Here's how the part is built. I have some questions about the finished solid (model axes, mm). Face numbers are marked on the shaded views. A direction names the side the tool comes from. Coordinates: 2 decimals unless noted, no trailing zeros. Order: outer loops, then holes, each group sorted by start corner. A loop starts at its lowest first (then second) coordinate and runs counter-clockwise, first axis right, second up. Notation, with made-up numbers: (-27, 54.5) - (29, 54.5) arc R19 cw to (29, 66.5) - close; hole circle Ø5 at (71.25, 87.25). An arc over 180 degrees is marked (long way). Answer in a Markdown table with one row per item. Add a question column.
Item 1: I want a section at A-A (z = 5.5). Please give me the cut outline in (x, y) (3 decimals).
Item 2: On a 3-axis mill with a long thin cutter (end or side, diameter ignored), from which of +Z, -Z, +X, -X, +Y, -Y can I reach the whole of each face in a straight line? I mean the marked faces 5, 6, 7 and 8. Say none if no direction works.
Item 3: Thinking about a two-plate mould opening in X: for the marked faces 1, 2, 3 and 4, which applies, +X half, -X half, draft (parallel to the pull), parting line (faces both ways), or undercut?
Item 4: Will these pins go through, and if not, where does the flat tip stop? pin 1 Ø4 at (x, z) = (19.5, 38) entering from -Y (3 decimals); pin 2 Ø2.5 at (y, z) = (-11, 63.5) entering from -X (3 decimals); pin 3 Ø18 at (x, y) = (-3, -55.5) entering from +Z (3 decimals).
Item 5: I want a section at B-B (y = -44.5). Please give me the cut outline in (x, z) (3 decimals).
Item 6: If I drill on line 1 along Y through (x, z) = (83.5, 46) (3 decimals); line 2 along X through (y, z) = (-36, 39) (3 decimals); line 3 along X through (y, z) = (-48, -2) (3 decimals), over which ranges is the centre line in solid material (lowest first)? Write a range as from..to.
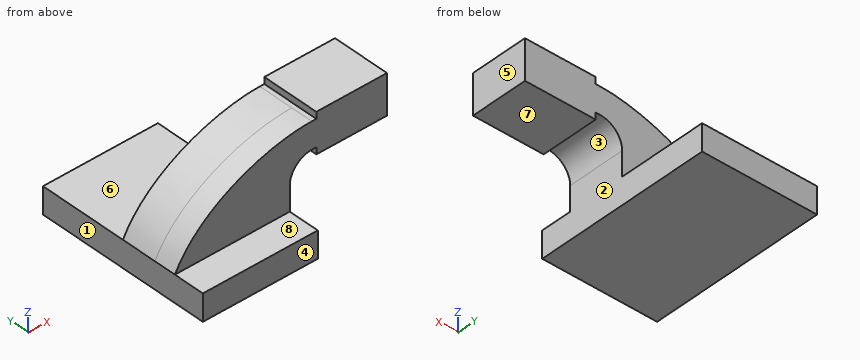
```python
from build123d import *

# Parameters (mm, degrees)
F1_DEPTH = 63.5
F0_W     = 25.4
F0_H     = 19.05
F0_H_2   = 4.7498
F0_H_3   = 4.7752
F2_DEPTH = 25.4
F3_DEPTH = 15.875


with BuildPart() as f1:
    # F0 (on Front) → F1 (new body, symmetric)
    with BuildSketch(Plane.XZ):
        Polygon((-41.275, -9.525), (41.275, -9.525), (41.275, 9.525), (22.225, 9.525), (-41.275, 9.525), align=None)
    extrude(amount=F1_DEPTH, both=True)

    # F0 (on Front) → F2 (join)
    with BuildSketch(Plane.XZ):
        Polygon((-41.275, -9.525), (41.275, -9.525), (41.275, 9.525), (22.225, 9.525), (-41.275, 9.525), align=None)
        with BuildLine():
            Line((22.225, 9.525), (41.275, 9.525))
            Line((41.275, 9.525), (41.275, 27.0002))
            ThreePointArc((41.275, 27.0002), (45.9246798487, 38.2255201513), (57.15, 42.8752))
            Line((57.15, 42.8752), (60.325, 42.8752))
            Line((60.325, 42.8752), (60.325, 61.9252))
            Line((60.325, 61.9252), (57.15, 61.9252))
            ThreePointArc((57.15, 61.9252), (32.4542956671, 51.6959043329), (22.225, 27.0002))
            Line((22.225, 27.0002), (22.225, 9.525))
        make_face()
        with BuildLine():
            add(Edge.make_bspline(
                [(-41.275, 9.525), (-23.4616156667, 44.3730577827), (24.9917246401, 62.0542801917), (57.15, 61.9252)],
                knots=[0, 0, 0, 0, 111.5045361635, 111.5045361635, 111.5045361635, 111.5045361635], degree=3))
            Line((-41.275, 9.525), (22.225, 9.525))
            Line((22.225, 9.525), (22.225, 27.0002))
            ThreePointArc((22.225, 27.0002), (32.4542956671, 51.6959043329), (57.15, 61.9252))
        make_face()
        with Locations((73.025, 52.4002)):
            Rectangle(F0_W, F0_H)
        with Locations((73.025, 64.3001)):
            Rectangle(F0_W, F0_H_2)
        with Locations((73.025, 40.4876)):
            Rectangle(F0_W, F0_H_3)
        Polygon((85.725, 66.675), (85.725, 61.9252), (85.725, 42.8752), (85.725, 38.1), (111.125, 38.1), (111.125, 66.675), align=None)
    extrude(amount=F2_DEPTH)

    # F0 (on Front) + F2_face (on face) → F3 (join)
    with BuildSketch(Plane.XZ):
        Polygon((-41.275, -9.525), (41.275, -9.525), (41.275, 9.525), (22.225, 9.525), (-41.275, 9.525), align=None)
        with BuildLine():
            Line((22.225, 9.525), (41.275, 9.525))
            Line((41.275, 9.525), (41.275, 27.0002))
            ThreePointArc((41.275, 27.0002), (45.9246798487, 38.2255201513), (57.15, 42.8752))
            Line((57.15, 42.8752), (60.325, 42.8752))
            Line((60.325, 42.8752), (60.325, 61.9252))
            Line((60.325, 61.9252), (57.15, 61.9252))
            ThreePointArc((57.15, 61.9252), (32.4542956671, 51.6959043329), (22.225, 27.0002))
            Line((22.225, 27.0002), (22.225, 9.525))
        make_face()
        with BuildLine():
            add(Edge.make_bspline(
                [(-41.275, 9.525), (-23.4616156667, 44.3730577827), (24.9917246401, 62.0542801917), (57.15, 61.9252)],
                knots=[0, 0, 0, 0, 111.5045361635, 111.5045361635, 111.5045361635, 111.5045361635], degree=3))
            Line((-41.275, 9.525), (22.225, 9.525))
            Line((22.225, 9.525), (22.225, 27.0002))
            ThreePointArc((22.225, 27.0002), (32.4542956671, 51.6959043329), (57.15, 61.9252))
        make_face()
        with Locations((73.025, 52.4002)):
            Rectangle(F0_W, F0_H)
        with Locations((73.025, 64.3001)):
            Rectangle(F0_W, F0_H_2)
        with Locations((73.025, 40.4876)):
            Rectangle(F0_W, F0_H_3)
        Polygon((85.725, 66.675), (85.725, 61.9252), (85.725, 42.8752), (85.725, 38.1), (111.125, 38.1), (111.125, 66.675), align=None)
    with BuildSketch(Plane(origin=(36.4198277408, -25.4, 38.4190839989), x_dir=(1, 0, 0), z_dir=(0, -1, 0))):
        with BuildLine():
            add(Edge.make_bspline(
                [(-77.6948277408, -28.8940839989), (-59.8814434075, 5.9539737837), (-11.4281031006, 23.6351961927), (20.7301722592, 23.5061160011)],
                knots=[0, 0, 0, 0, 111.5045361635, 111.5045361635, 111.5045361635, 111.5045361635], degree=3))
            Line((-77.6948277408, -28.8940839989), (4.8551722592, -28.8940839989))
            Line((4.8551722592, -28.8940839989), (4.8551722592, -11.4188839989))
            ThreePointArc((4.8551722592, -11.4188839989), (9.5048521079, -0.1935638476), (20.7301722592, 4.4561160011))
            Line((20.7301722592, 4.4561160011), (23.9051722592, 4.4561160011))
            Line((23.9051722592, 4.4561160011), (23.9051722592, -0.3190839989))
            Line((23.9051722592, -0.3190839989), (74.7051722592, -0.3190839989))
            Line((74.7051722592, -0.3190839989), (74.7051722592, 28.2559160011))
            Line((74.7051722592, 28.2559160011), (23.9051722592, 28.2559160011))
            Line((23.9051722592, 28.2559160011), (23.9051722592, 23.5061160011))
            Line((23.9051722592, 23.5061160011), (20.7301722592, 23.5061160011))
        make_face()
    extrude(amount=F3_DEPTH)


solid = f1.part
```
Values follow:
| question | item | result |
|---|---|---|
| 1 | outline | (-41.275, -63.5) - (41.275, -63.5) - (41.275, 63.5) - (-41.275, 63.5) - close |
| 2 | face 5 | +Z, -Z, +X, +Y, -Y |
| 2 | face 6 | +Z, +X, -X, +Y |
| 2 | face 7 | -Z, +X, +Y, -Y |
| 2 | face 8 | +Z, +X, -X, -Y |
| 3 | face 1 | -X half |
| 3 | face 2 | +X half |
| 3 | face 3 | undercut |
| 3 | face 4 | draft |
| 4 | pin 1 | stops at y = -41.275 |
| 4 | pin 2 | stops at x = 60.325 |
| 4 | pin 3 | stops at z = 9.525 |
| 5 | outline | (-41.275, -9.525) - (41.275, -9.525) - (41.275, 9.525) - (-41.275, 9.525) - close |
| 6 | line 1 | y = -41.275..0 |
| 6 | line 2 | x = -14.455..46.757, 60.325..111.125 |
| 6 | line 3 | x = -41.275..41.275 |
